```python
from build123d import *

# Parameters (mm, degrees)
SKETCH013_W     = 25.15
SKETCH013_H     = 12.45
PAD001_DEPTH    = 5.9
SKETCH018_W     = 9.3
SKETCH018_H     = 9.3
POCKET008_DEPTH = 1.4
CHAMFER_SIZE    = 0.8
PAD003_DEPTH    = 3
SKETCH007_W     = 6
SKETCH007_H     = 3
PAD004_DEPTH    = 2.6
SKETCH008_R     = 1.5
PAD005_DEPTH    = 2
FILLET004_R     = 0.5
CHAMFER003_SIZE = 1.3
FILLET003_R     = 1.5
FILLET002_R     = 1
SKETCH009_W     = 6
SKETCH009_H     = 1.6
POCKET006_DEPTH = 1.8
SKETCH010_W     = 6
SKETCH010_H     = 1.6
POCKET007_DEPTH = 1.8
SKETCH014_W     = 1.6
SKETCH014_H     = 6
POCKET005_DEPTH = 1.8


with BuildPart() as part:
    # Sketch013 → Pad001 (new body)
    with BuildSketch(Plane.XZ):
        Rectangle(SKETCH013_W, SKETCH013_H)
    extrude(amount=PAD001_DEPTH)

    # Sketch018 (on Face6 of Pad001) → Pocket008 (cut)
    with BuildSketch(Plane.XZ.offset(5.9)):
        with Locations((-6.35, 0)):
            Rectangle(SKETCH018_W, SKETCH018_H)
        with Locations((6.35, 0)):
            Rectangle(SKETCH018_W, SKETCH018_H)
    extrude(amount=-POCKET008_DEPTH, mode=Mode.SUBTRACT)

    # Chamfer
    chamfer_edges = [part.edges().sort_by_distance(p)[0] for p in [
        (-6.35, -5.9, 4.65),
        (-11, -5.9, 0),
        (-6.35, -5.9, -4.65),
        (-1.7, -5.9, 0),
        (1.7, -5.9, 0),
        (6.35, -5.9, 4.65),
        (11, -5.9, 0),
        (6.35, -5.9, -4.65),
    ]]
    chamfer(chamfer_edges, length=CHAMFER_SIZE)

    # Sketch015 (on Face18 of Chamfer) → Pad003 (join)
    with BuildSketch(Plane(origin=(0, 0, 0), x_dir=(1, 0, 0), z_dir=(0, 1, 0))):
        Polygon((12.575, -4.315), (12.575, -6.225), (10.945, -6.225), (10.945, -5.425), (11.775, -5.425), (11.775, -4.315), align=None)
        Polygon((-10.945, -6.225), (-12.575, -6.225), (-12.575, -4.315), (-11.775, -4.315), (-11.775, -5.425), (-10.945, -5.425), align=None)
        Polygon((12.575, 4.315), (12.575, 6.225), (10.945, 6.225), (10.945, 5.425), (11.775, 5.425), (11.775, 4.315), align=None)
        Polygon((-11.775, 4.315), (-11.775, 5.425), (-10.945, 5.425), (-10.945, 6.225), (-12.575, 6.225), (-12.575, 4.315), align=None)
    extrude(amount=PAD003_DEPTH)

    # Sketch007 (on Face19 of Pad003) → Pad004 (join)
    with BuildSketch(Plane(origin=(0, 0, 0), x_dir=(1, 0, 0), z_dir=(0, 1, 0))):
        with Locations((-6.2875, 4.725)):
            Rectangle(SKETCH007_W, SKETCH007_H)
        with Locations((6.2875, 4.725)):
            Rectangle(SKETCH007_W, SKETCH007_H)
        with Locations((-6.2875, -4.725)):
            Rectangle(SKETCH007_W, SKETCH007_H)
        with Locations((6.2875, -4.725)):
            Rectangle(SKETCH007_W, SKETCH007_H)
    extrude(amount=PAD004_DEPTH)

    # Sketch008 (on Face19 of Pad004) → Pad005 (join)
    with BuildSketch(Plane(origin=(0, 0, 0), x_dir=(1, 0, 0), z_dir=(0, 1, 0))):
        Circle(SKETCH008_R)
    extrude(amount=PAD005_DEPTH)

    # Fillet004
    fillet004_edges = [part.edges().sort_by_distance(p)[0] for p in [
        (-1.5, 2, 0),
    ]]
    fillet(fillet004_edges, radius=FILLET004_R)

    # Chamfer003
    chamfer003_edges = [part.edges().sort_by_distance(p)[0] for p in [
        (6.2875, 2.6, -6.225),
        (-6.2875, 2.6, -6.225),
        (6.2875, 2.6, 6.225),
        (-6.2875, 2.6, 6.225),
    ]]
    chamfer(chamfer003_edges, length=CHAMFER003_SIZE)

    # Fillet003
    fillet003_edges = [part.edges().sort_by_distance(p)[0] for p in [
        (-6.2875, 2.6, 4.925),
        (6.2875, 2.6, 4.925),
        (-6.2875, 2.6, -4.925),
        (6.2875, 2.6, -4.925),
    ]]
    fillet(fillet003_edges, radius=FILLET003_R)

    # Fillet002
    fillet002_edges = [part.edges().sort_by_distance(p)[0] for p in [
        (6.2875, 1.3, -6.225),
        (-6.2875, 1.3, -6.225),
        (6.2875, 1.3, 6.225),
        (-6.2875, 1.3, 6.225),
    ]]
    fillet(fillet002_edges, radius=FILLET002_R)

    # Sketch009 (on Face22 of Fillet002) → Pocket006 (cut)
    with BuildSketch(Plane(origin=(0, 0, 3.225), x_dir=(1, 0, 0), z_dir=(0, 0, -1))):
        with Locations((-6.2875, -0.8)):
            Rectangle(SKETCH009_W, SKETCH009_H)
    extrude(amount=-POCKET006_DEPTH, mode=Mode.SUBTRACT)

    # Sketch010 (on Face25 of Pocket006) → Pocket007 (cut)
    with BuildSketch(Plane(origin=(0, 0, 3.225), x_dir=(1, 0, 0), z_dir=(0, 0, -1))):
        with Locations((6.2875, -0.8)):
            Rectangle(SKETCH010_W, SKETCH010_H)
    extrude(amount=-POCKET007_DEPTH, mode=Mode.SUBTRACT)

    # Sketch014 (on DatumPlane) → Pocket005 (cut)
    with BuildSketch(Plane(origin=(0, 1.3, -3.225), x_dir=(0, 1, 0), z_dir=(0, 0, 1))):
        with Locations((-0.5, 6.2875)):
            Rectangle(SKETCH014_W, SKETCH014_H)
        with Locations((-0.5, -6.2875)):
            Rectangle(SKETCH014_W, SKETCH014_H)
    extrude(amount=-POCKET005_DEPTH, mode=Mode.SUBTRACT)


solid = part.part
```
Model file for the job. Use its own axes, mm. A direction names the side the tool comes from. Round coordinates to 2 decimals unless told otherwise and drop trailing zeros. Order: outer loops, then holes, each group sorted by start corner. A loop starts at its lowest first (then second) coordinate and runs counter-clockwise, first axis right, second up. Notation, with made-up numbers: (43, -9) -> (101, -9) arc R16 ccw to (101, 21) -> close; hole circle Ø2 at (-12.75, 4). An arc over 180 degrees is marked (long way). Use one line per item in the form item = value.
Item 1: Flat gauge pins, fed straight in: pin 1 Ø1 at (x, z) = (4.5, 2) entering from -Y; pin 2 Ø4 at (x, z) = (-7.5, 1.5) entering from +Y; pin 3 Ø1.4 at (x, z) = (6.5, -4.5) entering from -Y; pin 4 Ø3 at (y, z) = (0.5, 2) entering from +X (3 decimals). Where does each tip first touch, or does it go through?
Returned:
pin_1 = -4.5
pin_2 = 2.6
pin_3 = -5.65
pin_4 = 12.575
Item 2: Drill centre lines: line 1 (X direction, y = 1.25, z = -5.5) (1 decimal); line 2 (Y direction, x = -8.5, z = 4); line 3 (X direction, y = -5.5, z = -1.5) (3 decimals). Where is each one in solid material? Low to high.
Returned:
line_1 = -12.6 to -10.9, -9.3 to -3.3, 3.3 to 9.3, 10.9 to 12.6
line_2 = -4.5 to 0, 1.6 to 2.6
line_3 = -12.575 to -11.4, -1.3 to 1.3, 11.4 to 12.575
Item 3: Pull direction Z, two halves, no side cores. Call faces 4 (the face through (-6, 1, -5.025)), 5 (the face through (0, -3, 6.225)), 6 (the face through (0, 2, 0)): released by +Z, released by -Z, zero draft, split by the parting line, or undercut.
Returned:
face_4 = undercut
face_5 = released by +Z
face_6 = zero draft
Item 4: Tool access for faces 1 (the face through (0, 0, -3)), 2 (the face through (6.33, 2.48, 4.89)), 3 (the face through (-1.3, -5.5, -0.1)): list every direction of +Z, -Z, +X, -X, +Y, -Y with a clear straight run to the whole face (end or side of a thin tool).
Returned:
face_1 = none
face_2 = +Z, +Y
face_3 = -Y
Item 5: Cut at B-B, the plane x = -5.25. Write the cut outline in (y, z) (3 decimals).
Returned:
outline = (-5.9, -6.225) -> (0.886, -6.225) arc R1 ccw to (1.593, -5.932) -> (2.161, -5.364) arc R1.5 ccw to (2.6, -4.304) -> (2.6, -3.225) -> (1.6, -3.225) -> (1.6, -5.025) -> (0, -5.025) -> (0, 5.025) -> (1.6, 5.025) -> (1.6, 3.225) -> (2.6, 3.225) -> (2.6, 4.304) arc R1.5 ccw to (2.161, 5.364) -> (1.593, 5.932) arc R1 ccw to (0.886, 6.225) -> (-5.9, 6.225) -> (-5.9, 5.45) -> (-5.1, 4.65) -> (-4.5, 4.65) -> (-4.5, -4.65) -> (-5.1, -4.65) -> (-5.9, -5.45) -> close
Item 6: Cut at D-D, the plane x = 0. Write the cut outline in (y, z) (3 decimals).
Returned:
outline = (-5.9, -6.225) -> (0, -6.225) -> (0, -1.5) -> (1.5, -1.5) arc R0.5 ccw to (2, -1) -> (2, 1) arc R0.5 ccw to (1.5, 1.5) -> (0, 1.5) -> (0, 6.225) -> (-5.9, 6.225) -> close
Item 7: Cut at C-C, the plane z = 0. Write the cut outline in (x, y) (3 decimals).
Returned:
outline = (-12.575, -5.9) -> (-11.8, -5.9) -> (-11, -5.1) -> (-11, -4.5) -> (-1.7, -4.5) -> (-1.7, -5.1) -> (-0.9, -5.9) -> (0.9, -5.9) -> (1.7, -5.1) -> (1.7, -4.5) -> (11, -4.5) -> (11, -5.1) -> (11.8, -5.9) -> (12.575, -5.9) -> (12.575, 0) -> (1.5, 0) -> (1.5, 1.5) arc R0.5 ccw to (1, 2) -> (-1, 2) arc R0.5 ccw to (-1.5, 1.5) -> (-1.5, 0) -> (-12.575, 0) -> close
Item 8: Cut at A-A, the plane z = 4. Write the cut outline in (x, y) (1 decimal).
Returned:
outline = (-12.6, -5.9) -> (-11.8, -5.9) -> (-11, -5.1) -> (-11, -4.5) -> (-1.7, -4.5) -> (-1.7, -5.1) -> (-0.9, -5.9) -> (0.9, -5.9) -> (1.7, -5.1) -> (1.7, -4.5) -> (11, -4.5) -> (11, -5.1) -> (11.8, -5.9) -> (12.6, -5.9) -> (12.6, 0) -> (-12.6, 0) -> close; (-9.3, 1.6) -> (-3.3, 1.6) -> (-3.3, 2.6) -> (-9.3, 2.6) -> close; (3.3, 1.6) -> (9.3, 1.6) -> (9.3, 2.6) -> (3.3, 2.6) -> close
